from build123d import *

# Parameters (mm, degrees)
SKETCH048_W         = 40
SKETCH048_H         = 24
PAD013_DEPTH        = 3
HOLE020_D           = 2.8
HOLE020_DEPTH       = 25
HOLE020_CBORE_D     = 6
HOLE020_CBORE_DEPTH = 1.5
SKETCH050_R         = 6.7
HOLE021_DEPTH       = 25
FILLET025_R         = 2


with BuildPart() as part:
    # Sketch048 → Pad013 (new body)
    with BuildSketch(Plane.XY):
        Rectangle(SKETCH048_W, SKETCH048_H)
    extrude(amount=PAD013_DEPTH)

    # Hole020
    with Locations(Plane.XY.offset(3)):
        with Locations((16.2, 8.2), (16.2, -8.2)):
            hole020 = CounterBoreHole(HOLE020_D / 2, HOLE020_CBORE_D / 2, HOLE020_CBORE_DEPTH, depth=HOLE020_DEPTH)

    # Mirrored023: Hole020 across Sketch049 V_Axis
    add(hole020.mirror(Plane(origin=(0, 0, 3), x_dir=(0, 0, 1), z_dir=(1, 0, 0))), mode=Mode.SUBTRACT)

    # Sketch050 (on Face5 of Mirrored023) → Hole021 (cut)
    with BuildSketch(Plane.XY.offset(3)):
        with Locations((7.5, 0)):
            Circle(SKETCH050_R)
    hole021 = extrude(amount=-HOLE021_DEPTH, mode=Mode.SUBTRACT)

    # Mirrored024: Hole021 across Sketch050 V_Axis
    add(hole021.mirror(Plane(origin=(0, 0, 3), x_dir=(0, 0, 1), z_dir=(1, 0, 0))), mode=Mode.SUBTRACT)

    # Fillet025
    fillet025_edges = [part.edges().sort_by_distance(p)[0] for p in [
        (20, 12, 1.5),
        (-20, 12, 1.5),
        (-20, -12, 1.5),
        (20, -12, 1.5),
    ]]
    fillet(fillet025_edges, radius=FILLET025_R)


solid = part.part
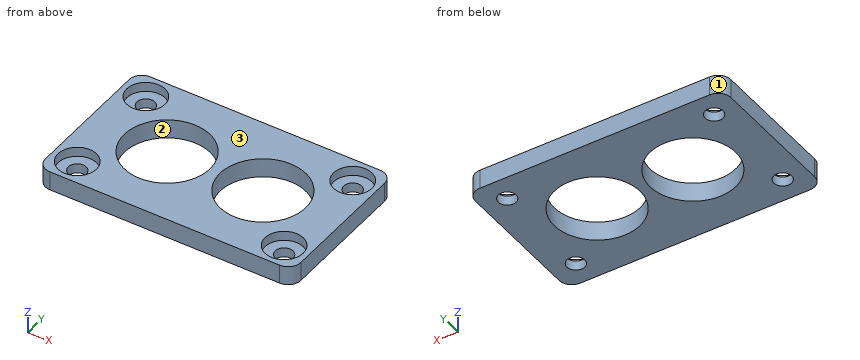
CAD build for the part. Positions are in the model's coordinates, mm. Face numbers are marked on the shaded views. Coordinates: 2 decimals unless noted, no trailing zeros. Write each loop counter-clockwise with the first axis right and the second up, starting at its lowest first coordinate (ties: lowest second). Pieces come first, ordered by that corner, then holes. Notation, with made-up numbers: (74.5, 68) - (96.5, 68) arc R17 cw to (96.5, 97) - close; hole circle Ø2 at (-13.75, -18.75). An arc over 180 degrees is marked (long way). Use a Markdown table: item, result. Add a question column.
Item 1: Mould opens along X. For the marked faces 1, 2 and 3 say: pulls with the +X half, pulls with the -X half, needs draft (parallel to the pull), parting line crosses it, or undercut.
Item 2: Band-saw the part on A-A, the plane y = 0. Give the cut face in (x, z).
Item 3: Drill centre lines: L1, parallel to Y at x = -16.2, z = 2; L2, parallel to Y at x = -16.2, z = 0.4; L3, parallel to Y at x = -7.5, z = 1.05. Where is each one in solid material? Low to high. Write a range as from..to.
Item 4: Band-saw the part on C-C, the plane z = 2. Give the cut face in (x, y).
Item 5: Band-saw the part on D-D, the plane x = 7.5. Give the cut face in (y, z).
Item 6: Flat gauge pins, fed straight in: pin 1 (4.5 mm diameter, centred on x = -16.2, y = 8.2, fed in from +Z); pin 2 (3 mm diameter, centred on x = 6.5, y = 5, fed in from -Z); pin 3 (9.5 mm diameter, centred on x = 16.2, y = 8.2, fed in from +Z). Where does each tip first touch, or does it go through?
Item 7: Band-saw the part on B-B, the plane x = -16.2. Give the cut face in (y, z), and give its area (3 significant figures).
Numbers:
| question | item | result |
|---|---|---|
| 1 | face 1 | pulls with the -X half |
| 1 | face 2 | undercut |
| 1 | face 3 | needs draft |
| 2 | outline | (-20, 0) - (-14.2, 0) - (-14.2, 3) - (-20, 3) - close; (-0.8, 0) - (0.8, 0) - (0.8, 3) - (-0.8, 3) - close; (14.2, 0) - (20, 0) - (20, 3) - (14.2, 3) - close |
| 3 | L1 | -12..-11.2, -5.2..5.2, 11.2..12 |
| 3 | L2 | -12..-9.6, -6.8..6.8, 9.6..12 |
| 3 | L3 | -12..-6.7, 6.7..12 |
| 4 | outline | (-20, -10) arc R2 ccw to (-18, -12) - (18, -12) arc R2 ccw to (20, -10) - (20, 10) arc R2 ccw to (18, 12) - (-18, 12) arc R2 ccw to (-20, 10) - close; hole circle Ø6 at (-16.2, -8.2); hole circle Ø6 at (-16.2, 8.2); hole circle Ø13.4 at (-7.5, 0); hole circle Ø13.4 at (7.5, 0); hole circle Ø6 at (16.2, -8.2); hole circle Ø6 at (16.2, 8.2) |
| 5 | outline | (-12, 0) - (-6.7, 0) - (-6.7, 3) - (-12, 3) - close; (6.7, 0) - (12, 0) - (12, 3) - (6.7, 3) - close |
| 6 | pin 1 | z = 1.5 |
| 6 | pin 2 | through |
| 6 | pin 3 | z = 3 |
| 7 | outline | (-12, 0) - (-9.6, 0) - (-9.6, 1.5) - (-11.2, 1.5) - (-11.2, 3) - (-12, 3) - close; (-6.8, 0) - (6.8, 0) - (6.8, 1.5) - (5.2, 1.5) - (5.2, 3) - (-5.2, 3) - (-5.2, 1.5) - (-6.8, 1.5) - close; (9.6, 0) - (12, 0) - (12, 3) - (11.2, 3) - (11.2, 1.5) - (9.6, 1.5) - close |
| 7 | area | 45.6 mm2 |
